Autodesk Inventor part; units mm, degrees
ref_plane "YZ Plane" through (0, 0, 0) normal (1, 0, 0) x (0, 1, 0)
ref_plane "XZ Plane" through (0, 0, 0) normal (0, 1, 0) x (-1, 0, 0)
ref_plane "XY Plane" through (0, 0, 0) normal (0, 0, 1) x (1, 0, 0)
sketch "Sketch4" plane through (0, 0, 0) normal (0, 0, 1) x (1, 0, 0)
  line L0 (-21.5, 10.75) -> (0, 10.75)
  line L1 (0, 10.75) -> (0, -10.75)
  line L2 (0, -10.75) -> (-21.5, -10.75)
  line L3 (-21.5, -10.75) -> (-21.5, 10.75)
  circle A0 centre (-10.75, 0) radius 2.2
  point P0 (0, 0)
  point P1 (-21.5, 0)
  point P2 (0, 0)
  point P3 (-10.75, 10.75)
  dimension "d12" = 21.5
  dimension "d13" = 21.5
  dimension "d14" = 4.4
extrude "Extrusion4" add sketch "Sketch4" along normal blind 1.75
sketch "Sketch5" plane through (0, 0, 1.75) normal (0, 0, 1) x (1, 0, 0)
  circle A0 centre (-10.75, 0) radius 2.2
  circle A1 centre (-10.75, 0) radius 6.7
  point P0 (0, 0)
  dimension "d17" = 13.4
extrude "Extrusion5" add sketch "Sketch5" along normal blind 1.65
draft "FaceDraft2" angle 45 pull direction (0, 0, 1) faces at (-4.1368, -1.0748, 2.85) fixed edges at (-17.45, 0, 1.75)
sketch "Sketch6" plane through (-10.75, 0, 3.4) normal (0, 0, 1) x (1, 0, 0)
  circle A0 centre (0, 0) radius 2.2
  circle A1 centre (0, 0) radius 5.05
  line L0 (2.1362, -3.7) -> (-2.1362, -3.7)
  line L1 (-2.1362, -3.7) -> (-4.2724, 0)
  line L2 (-4.2724, 0) -> (-2.1362, 3.7)
  line L3 (-2.1362, 3.7) -> (2.1362, 3.7)
  line L4 (2.1362, 3.7) -> (4.2724, 0)
  line L5 (4.2724, 0) -> (2.1362, -3.7)
  line L6 (-10.75, 10.75) -> (10.75, 10.75)
  point P0 (10.75, 0)
  dimension "d21" = 7.4
extrude "Extrusion6" cut sketch "Sketch6" against normal blind 2.4 contours L0 L1 L2 L3 L4 L5
mirror "Mirror1" about plane through (0, 10.75, 0) normal (1, 0, 0) of "Extrusion4", "FaceDraft2", "Extrusion5", "Extrusion6"
properties part number "bracket_plastictube"
Work out the finished part from the listing and answer in its coordinate system (mm). A direction names the side the tool comes from. Give positions to 0.01 mm unless a question says otherwise; leave off trailing zeros. Order: outer loops, then holes, each group sorted by start corner. A loop starts at its lowest first (then second) coordinate and runs counter-clockwise, first axis right, second up. Notation, with made-up numbers: (55, 85) - (112, 85) arc R4 cw to (112, 92) - close; hole circle Ø3 at (14.5, 86). An arc over 180 degrees is marked (long way). One line per item, written item: value. Start each with the question number.
1. Section A-A, the plane x = -10.75 is taken. Write down the section's boundary in (y, z), then the cut area to 3 significant figures.
2. For a pull along X with two mould halves and no side action, classify faces 1 (the face through (21.5, 0, 1)), 2 (the face through (0, 0, 0)), 3 (the face through (0, 0, 1.75)) as released by +X, released by -X, zero draft, split by the parting line, or undercut.
3. Consider line 1 (Y direction, x = 10.75, z = 0.8); line 2 (X direction, y = -3.25, z = 1.95); line 3 (X direction, y = 3, z = 2.8). Determine where each line is inside the solid, lowest interval first.
4. Which of the six approach directions +Z, -Z, +X, -X, +Y, -Y give full straight-line access (tool end or side, diameter ignored) to faces 4 (the face through (-8.7, 0.8, 0.5)), 5 (the face through (-7.53, -1.82, 2.22))?
5. Each of these flat-tipped pins is pushed along its axis until it touches: pin 1 Ø12 at (x, y) = (6, 3.5) entering from -Z; pin 2 Ø2.5 at (x, y) = (-10.75, 0) entering from -Z; pin 3 Ø6 at (x, y) = (10.5, 0) entering from +Z; pin 4 Ø1 at (x, y) = (2.5, -3) entering from +Z. Where does it stop, or does it pass through?
6. Section C-C, the plane y = 0.5 is taken. Count the separate pieces of the cut face and the enclosed holes in it, then the cut area to 3 significant figures.
7. Section B-B, the plane y = -7.5 is taken. Write down the section's boundary in (x, z).
Filled sheet:
1. outline: (-10.75, 0) - (-2.2, 0) - (-2.2, 1) - (-3.7, 1) - (-3.7, 3.4) - (-5.05, 3.4) - (-6.7, 1.75) - (-10.75, 1.75) - close; (2.2, 0) - (10.75, 0) - (10.75, 1.75) - (6.7, 1.75) - (5.05, 3.4) - (3.7, 3.4) - (3.7, 1) - (2.2, 1) - close
1. area: 34.9 mm²
2. face 1: released by +X
2. face 2: zero draft
2. face 3: undercut
3. line 1: -10.75 to -2.2, 2.2 to 10.75
3. line 2: -16.38 to -13.15, -8.35 to -5.12, 5.12 to 8.35, 13.15 to 16.38
3. line 3: -15.54 to -13.29, -8.21 to -5.96, 5.96 to 8.21, 13.29 to 15.54
4. face 4: +Z, -Z
4. face 5: +Z
5. pin 1: z = 0
5. pin 2: through
5. pin 3: z = 1
5. pin 4: z = 1.75
6. separate pieces: 3
6. enclosed holes: 0
6. area: 67.1 mm²
7. outline: (-21.5, 0) - (21.5, 0) - (21.5, 1.75) - (-21.5, 1.75) - close
